from build123d import *

# Parameters (mm, degrees)
SKETCH1_W                                           = 38.1
SKETCH1_H                                           = 43.18
BOSS_EXTRUDE1_DEPTH                                 = 17.78
SKETCH2_R                                           = 10.795
CUT_EXTRUDE1_DEPTH                                  = 61.26815743
CBORE_FOR_6_BINDING_HEAD_MACHINE_SCREW1_D           = 3.7973
CBORE_FOR_6_BINDING_HEAD_MACHINE_SCREW1_CBORE_D     = 7.9375
CBORE_FOR_6_BINDING_HEAD_MACHINE_SCREW1_CBORE_DEPTH = 2.2098


with BuildPart() as part:
    # Sketch1 → Boss-Extrude1 (new body)
    with BuildSketch(Plane.XY):
        with Locations((19.05, 21.59)):
            Rectangle(SKETCH1_W, SKETCH1_H)
    extrude(amount=BOSS_EXTRUDE1_DEPTH)

    # Sketch2 → Cut-Extrude1 (cut, through all)
    with BuildSketch(Plane.ZY):
        with Locations((17.78, 21.59)):
            Circle(SKETCH2_R)
    extrude(amount=-CUT_EXTRUDE1_DEPTH, mode=Mode.SUBTRACT)

    # CBORE for #6 Binding Head Machine Screw1 (through all)
    with Locations(Plane(origin=(28.701956409, 37.846, 0), x_dir=(-1, 0, 0), z_dir=(0, 0, -1))):
        with Locations((0, 0), (19.049956409, -0.040753052), (0.253956409, -32.99093936), (19.297934909, -32.512)):
            CounterBoreHole(CBORE_FOR_6_BINDING_HEAD_MACHINE_SCREW1_D / 2, CBORE_FOR_6_BINDING_HEAD_MACHINE_SCREW1_CBORE_D / 2, CBORE_FOR_6_BINDING_HEAD_MACHINE_SCREW1_CBORE_DEPTH)


solid = part.part
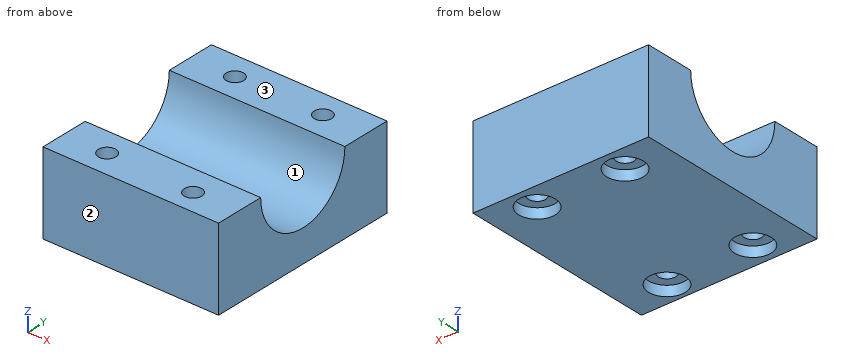
The listing builds one solid part. Answer for the finished solid, in the listing's coordinates (mm). Face numbers are marked on the shaded views. Round coordinates to 2 decimals unless told otherwise and drop trailing zeros. Write each loop counter-clockwise with the first axis right and the second up, starting at its lowest first coordinate (ties: lowest second). Pieces come first, ordered by that corner, then holes. Notation, with made-up numbers: M 53.25,89.5 L 58.25,89.5 A31 ccw 58.25,128.5 Z; hole C 46.5,43.25 d1. An arc over 180 degrees is marked long. Write each question's results on one line, items separated by ' | '. Start each with the question number.
(1) The part is cut by section C-C, the plane y = 21.59. Write down the section's boundary in (x, z) (3 decimals), and give its area (3 significant figures).
(2) The part is cut by section B-B, the plane x = 29.5. Write down the section's boundary in (y, z) (1 decimal).
(3) Determine the mould class of the marked faces 1, 2 and 3 for opening direction Y: +Y half, -Y half, draft (parallel to the pull), parting line (faces both ways), or undercut.
(4) Each of these flat-tipped pins is pushed along its axis until it touches: P1, Ø5, axis at x = 28, y = 16, coming from the +Z side; P2, Ø4, axis at x = 28, y = 36.5, coming from the -Z side. Where does it stop, or does it pass through?
(5) The part is cut by section D-D, the plane z = 5. Write down the section's boundary in (x, y).
(6) The part is cut by section A-A, the plane z = 9.25. Write down the section's boundary in (x, y).
(7) Find the intervals of material crossed by line 1 (Y direction, x = 9, z = 14); line 2 (Y direction, x = 8.5, z = 9); line 3 (X direction, y = 4.5, z = 12.25), in increasing order.
Worked answers:
1) outline: M 0,0 L 38.1,0 L 38.1,6.985 L 0,6.985 Z | area: 266 mm²
2) outline: M 0,0 L 1,0 L 1,2.2 L 3.3,2.2 L 3.3,17.8 L 0,17.8 Z; M 6.4,2.2 L 8.7,2.2 L 8.7,0 L 34,0 L 34,2.2 L 36.1,2.2 L 36.1,17.8 L 32.4,17.8 A10.8 cw 10.8,17.8 L 6.4,17.8 Z; M 39.6,2.2 L 41.7,2.2 L 41.7,0 L 43.2,0 L 43.2,17.8 L 39.6,17.8 Z
3) face 1: undercut | face 2: -Y half | face 3: draft
4) P1: stops at z = 10.63 | P2: stops at z = 2.21
5) outline: M 0,0 L 38.1,0 L 38.1,43.18 L 0,43.18 Z; hole C 9.4,5.33 d3.8; hole C 9.65,37.81 d3.8; hole C 28.45,4.86 d3.8; hole C 28.7,37.85 d3.8
6) outline: M 0,0 L 38.1,0 L 38.1,14.97 L 0,14.97 Z; M 0,28.21 L 38.1,28.21 L 38.1,43.18 L 0,43.18 Z; hole C 9.4,5.33 d3.8; hole C 9.65,37.81 d3.8; hole C 28.45,4.86 d3.8; hole C 28.7,37.85 d3.8
7) line 1: y = 0 to 3.48, 7.19 to 11.48, 31.7 to 36.02, 39.59 to 43.18 | line 2: y = 0 to 3.66, 7 to 15.31, 27.87 to 36.3, 39.31 to 43.18 | line 3: x = 0 to 7.7, 11.11 to 26.58, 30.31 to 38.1
